from build123d import *

# Parameters (mm, degrees)
F0_W     = 350
F0_H     = 150
F0_R     = 4.25
F0_R_2   = 11
F0_R_3   = 7.5
F0_W_2   = 69
F0_H_2   = 21.5
F1_DEPTH = 2.5


with BuildPart() as f1:
    # F0 (on Front) → F1 (new body)
    with BuildSketch(Plane.XZ):
        Rectangle(F0_W, F0_H)
        with Locations((-148.5, -31)):
            Circle(F0_R, mode=Mode.SUBTRACT)
        with Locations((-41.5, -31)):
            Circle(F0_R, mode=Mode.SUBTRACT)
        with Locations((-115, 0)):
            Circle(F0_R_2, mode=Mode.SUBTRACT)
        with Locations((-148.5, 31)):
            Circle(F0_R, mode=Mode.SUBTRACT)
        with Locations((-75, 0)):
            Circle(F0_R_3, mode=Mode.SUBTRACT)
        with Locations((-41.5, 31)):
            Circle(F0_R, mode=Mode.SUBTRACT)
        with Locations((80.5, 14.25)):
            Rectangle(F0_W_2, F0_H_2, mode=Mode.SUBTRACT)
    extrude(amount=F1_DEPTH)


solid = f1.part
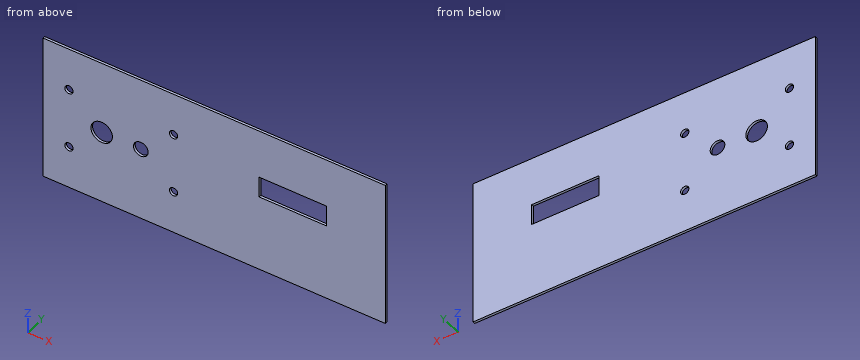
The model under review builds one solid part; all positions refer to its coordinate system, in mm. Round coordinates to 2 decimals unless told otherwise and drop trailing zeros. Order: outer loops, then holes, each group sorted by start corner. A loop starts at its lowest first (then second) coordinate and runs counter-clockwise, first axis right, second up. Notation, with made-up numbers: (67.25, 55.25) -> (117.25, 55.25) arc R15 cw to (117.25, 78.25) -> close; hole circle Ø1 at (52.5, 59). An arc over 180 degrees is marked (long way). Use CSV: the item, a comma, the result in double quotes. Start each with the question number.
(1) Wall thickness on probe 1 along Z at (x, y) = (85, -0.85); probe 2 along X at (y, z) = (-0.35, 20); probe 3 along Z at (x, y) = (-115, -1.25): over which ranges is each line inside the solid? List them lowest first. Write a range as from..to.
(2) Consider section C-C on x = -75. Write out the cut boundary in (y, z), and give its area (4 significant figures).
(3) Consider section A-A on x = -115. Write out the cut boundary in (y, z).
(4) Consider section B-B on z = 0. Write out the cut boundary in (x, y), and give its area (4 significant figures).
(5) Consider section D-D on z = -31. Write out the cut boundary in (x, y), and give its area (4 significant figures).
(6) Insertion check: pin 1 (19.5 mm diameter, centred on x = -75, z = 0, fed in from +Y). The pin has a flat end and moves straight along its axis. Give the tip position at first contact, or say it passes through.
Responses:
1,probe 1,"-75..3.5, 25..75"
1,probe 2,"-175..46, 115..175"
1,probe 3,"-75..-11, 11..75"
2,outline,"(-2.5, -75) -> (0, -75) -> (0, -7.5) -> (-2.5, -7.5) -> close; (-2.5, 7.5) -> (0, 7.5) -> (0, 75) -> (-2.5, 75) -> close"
2,area,"337.5 mm²"
3,outline,"(-2.5, -75) -> (0, -75) -> (0, -11) -> (-2.5, -11) -> close; (-2.5, 11) -> (0, 11) -> (0, 75) -> (-2.5, 75) -> close"
4,outline,"(-175, -2.5) -> (-126, -2.5) -> (-126, 0) -> (-175, 0) -> close; (-104, -2.5) -> (-82.5, -2.5) -> (-82.5, 0) -> (-104, 0) -> close; (-67.5, -2.5) -> (175, -2.5) -> (175, 0) -> (-67.5, 0) -> close"
4,area,"782.5 mm²"
5,outline,"(-175, -2.5) -> (-152.75, -2.5) -> (-152.75, 0) -> (-175, 0) -> close; (-144.25, -2.5) -> (-45.75, -2.5) -> (-45.75, 0) -> (-144.25, 0) -> close; (-37.25, -2.5) -> (175, -2.5) -> (175, 0) -> (-37.25, 0) -> close"
5,area,"832.5 mm²"
6,pin 1,"y = 0"
